```python
from build123d import *

# Parameters (mm, degrees)
CROQUIS1_R                                           = 12.5
SALIENTE_EXTRUIR1_DEPTH                              = 3.5
TALADRO_DE_MARGEN_PARA_M31_D                         = 3.4
REFRENTADO_PARA_TORNILLO_TAP_N_CON_CABEZ_D           = 3.4
REFRENTADO_PARA_TORNILLO_TAP_N_CON_CABEZ_CSINK_D     = 6.72
REFRENTADO_PARA_TORNILLO_TAP_N_CON_CABEZ_CSINK_ANGLE = 90
SALIENTE_EXTRUIR2_START                              = -29
SALIENTE_EXTRUIR2_DEPTH                              = 29
SALIENTE_EXTRUIR3_DEPTH                              = 3.5
REFRENTADO_PARA_TORNILLO_CON_CABEZA_TRON_D           = 3.4
REFRENTADO_PARA_TORNILLO_CON_CABEZA_TRON_CBORE_D     = 7
REFRENTADO_PARA_TORNILLO_CON_CABEZA_TRON_CBORE_DEPTH = 2.4


with BuildPart() as part:
    # Croquis1 → Saliente-Extruir1 (new body)
    with BuildSketch(Plane(origin=(0, 0, 0), x_dir=(0, 0, -1), z_dir=(1, 0, 0))):
        with BuildLine():
            Line((-15, 40), (-15, 29.05666877))
            ThreePointArc((-15, 29.05666877), (0, -32.7), (15, 29.05666877))
            Line((15, 29.05666877), (15, 40))
            Line((15, 40), (32.5, 40))
            ThreePointArc((32.5, 40), (47.5, 55), (32.5, 70))
            Line((32.5, 70), (-32.5, 70))
            ThreePointArc((-32.5, 70), (-47.5, 55), (-32.5, 40))
            Line((-32.5, 40), (-15, 40))
        make_face()
        Circle(CROQUIS1_R, mode=Mode.SUBTRACT)
        with BuildLine():
            Line((-32.5, 67.5), (32.5, 67.5))
            ThreePointArc((32.5, 67.5), (45, 55), (32.5, 42.5))
            Line((32.5, 42.5), (-32.5, 42.5))
            ThreePointArc((-32.5, 42.5), (-45, 55), (-32.5, 67.5))
        make_face(mode=Mode.SUBTRACT)
    extrude(amount=SALIENTE_EXTRUIR1_DEPTH)

    # Taladro de margen para M31 (through all)
    with Locations(Plane(origin=(3.5, 0, 0), x_dir=(0, 0, -1), z_dir=(1, 0, 0))):
        with Locations((0, 29), (25.11473671, 14.5), (25.11473671, -14.5), (0, -29), (-25.11473671, -14.5), (-25.11473671, 14.5)):
            Hole(TALADRO_DE_MARGEN_PARA_M31_D / 2)

    # Refrentado para tornillo tapón con cabeza plana de clavija de M31 (through all)
    with Locations(Plane(origin=(3.5, 0, 0), x_dir=(0, 0, -1), z_dir=(1, 0, 0))):
        with Locations((12.374368671, 12.374368671), (-12.374368671, -12.374368671), (-12.374368671, 12.374368671), (12.374368671, -12.374368671)):
            CounterSinkHole(REFRENTADO_PARA_TORNILLO_TAP_N_CON_CABEZ_D / 2, REFRENTADO_PARA_TORNILLO_TAP_N_CON_CABEZ_CSINK_D / 2, counter_sink_angle=REFRENTADO_PARA_TORNILLO_TAP_N_CON_CABEZ_CSINK_ANGLE)

    # Croquis8 → Saliente-Extruir2 (add)
    with BuildSketch(Plane(origin=(3.5, 0, 0), x_dir=(0, 0, -1), z_dir=(1, 0, 0)).offset(SALIENTE_EXTRUIR2_START)):
        with BuildLine():
            Line((15, 40), (32.5, 40))
            ThreePointArc((32.5, 40), (47.5, 55), (32.5, 70))
            Line((32.5, 70), (-32.5, 70))
            ThreePointArc((-32.5, 70), (-47.5, 55), (-32.5, 40))
            Line((-32.5, 40), (-15, 40))
            Line((-15, 40), (15, 40))
        make_face()
        with BuildLine():
            Line((-32.5, 67.5), (32.5, 67.5))
            ThreePointArc((32.5, 67.5), (45, 55), (32.5, 42.5))
            Line((32.5, 42.5), (-32.5, 42.5))
            ThreePointArc((-32.5, 42.5), (-45, 55), (-32.5, 67.5))
        make_face(mode=Mode.SUBTRACT)
    extrude(amount=SALIENTE_EXTRUIR2_DEPTH)

    # Croquis12 → Saliente-Extruir3 (add)
    with BuildSketch(Plane.ZY.offset(25.5)):
        with BuildLine():
            Line((32.5, 42.5), (-32.5, 42.5))
            ThreePointArc((-32.5, 42.5), (-45, 55), (-32.5, 67.5))
            Line((-32.5, 67.5), (32.5, 67.5))
            ThreePointArc((32.5, 67.5), (45, 55), (32.5, 42.5))
        make_face()
    extrude(amount=-SALIENTE_EXTRUIR3_DEPTH)

    # Refrentado para tornillo con cabeza troncocónica de M31 (through all)
    with Locations(Plane.ZY.offset(25.5)):
        with Locations((-22.5, 55), (22.5, 55)):
            CounterBoreHole(REFRENTADO_PARA_TORNILLO_CON_CABEZA_TRON_D / 2, REFRENTADO_PARA_TORNILLO_CON_CABEZA_TRON_CBORE_D / 2, REFRENTADO_PARA_TORNILLO_CON_CABEZA_TRON_CBORE_DEPTH)


solid = part.part
```
The listing builds one solid part. Answer for the finished solid, in the listing's coordinates (mm). A direction names the side the tool comes from. Coordinates: 2 decimals unless noted, no trailing zeros. Write each loop counter-clockwise with the first axis right and the second up, starting at its lowest first coordinate (ties: lowest second). Pieces come first, ordered by that corner, then holes. Notation, with made-up numbers: M 19,59.25 L 45,59.25 A9 cw 45,70.25 Z; hole C 51,76 d1. An arc over 180 degrees is marked long. Use a Markdown table: item, result. Add a question column.
1. Section D-D (y = 0) is taken. Give the vertices of the cut face in (x, z).
2. Which of the six approach directions +Z, -Z, +X, -X, +Y, -Y give full straight-line access (tool end or side, diameter ignored) to faces 4 (the flat face through (-23.1, 53, 22)), 5 (the flat face through (2, 35, 15)), 6 (the flat face through (2, 34, -15)), 7 (the cylindrical face through (-9, 55, -45))?
3. Given P1, Ø3, axis at x = 1.5, y = 32, coming from the +Z side; P2, Ø3, axis at y = 12.37, z = 12.37, coming from the +X side; P3, Ø13, axis at x = -5, z = -9, coming from the -Y side; P4, Ø5.5, axis at y = 14.5, z = 25.11, coming from the -X side, each flat-ended and moving along its own axis, determine where each tip first touches the part or whether it passes through.
4. Section B-B (x = -20.5) is taken. Give the vertices of the cut face in (y, z).
5. Section C-C (z = 0) is taken. Give the vertices of the cut face in (x, y), plus the area to 3 significant figures.
6. Straight lines are drawn through the part: line 1 along Y through (x, z) = (-22.2, -22.5); line 2 along Z through (x, y) = (-22.25, 56.5); line 3 along Y through (x, z) = (-1, -12). For each, find the intervals that lie inside material, in ascending order. Write a range as [from, to].
7. Section A-A (y = 55) is taken. Give the vertices of the cut face in (x, z).
8. For a pull along Z with two mould halves and no side action, classify faces 1 (the flat face through (3.5, 19, 1)), 2 (the cylindrical face through (-24.32, 57.95, 24.38)), 3 (the cylindrical face through (-11.203, 55.33, 47.496)) as +Z half, -Z half, draft (parallel to the pull), parting line (faces both ways), or undercut.
Data:
| question | item | result |
|---|---|---|
| 1 | outline | M 0,-32.7 L 3.5,-32.7 L 3.5,-12.5 L 0,-12.5 Z; M 0,12.5 L 3.5,12.5 L 3.5,32.7 L 0,32.7 Z |
| 2 | face 4 | -X |
| 2 | face 5 | +Z, +X, -X |
| 2 | face 6 | -Z, +X, -X |
| 2 | face 7 | +X |
| 3 | P1 | stops at z = 15 |
| 3 | P2 | passes through |
| 3 | P3 | stops at y = -32.34 |
| 3 | P4 | stops at x = 0 |
| 4 | outline | M 40,-32.5 A15 ccw 70,-32.5 L 70,32.5 A15 ccw 40,32.5 Z; hole M 42.5,-32.5 A12.5 ccw 67.5,-32.5 L 67.5,32.5 A12.5 ccw 42.5,32.5 Z |
| 5 | outline | M -25.5,40 L 0,40 L 0,30.7 L 3.5,30.7 L 3.5,42.5 L -22,42.5 L -22,67.5 L 3.5,67.5 L 3.5,70 L -25.5,70 Z; M 0,-32.7 L 3.5,-32.7 L 3.5,-30.7 L 0,-30.7 Z; M 0,-27.3 L 3.5,-27.3 L 3.5,-12.5 L 0,-12.5 Z; M 0,12.5 L 3.5,12.5 L 3.5,27.3 L 0,27.3 Z |
| 5 | area | 376 mm2 |
| 6 | line 1 | y = [40, 53.3], [56.7, 70] |
| 6 | line 2 | z = [-47.42, -23.3], [-21.7, 21.7], [23.3, 47.42] |
| 6 | line 3 | y = [40, 42.5], [67.5, 70] |
| 7 | outline | M -25.5,-47.5 L 3.5,-47.5 L 3.5,-45 L -22,-45 L -22,-24.2 L -23.1,-24.2 L -23.1,-26 L -25.5,-26 Z; M -25.5,-19 L -23.1,-19 L -23.1,-20.8 L -22,-20.8 L -22,20.8 L -23.1,20.8 L -23.1,19 L -25.5,19 Z; M -25.5,26 L -23.1,26 L -23.1,24.2 L -22,24.2 L -22,45 L 3.5,45 L 3.5,47.5 L -25.5,47.5 Z |
| 8 | face 1 | draft |
| 8 | face 2 | undercut |
| 8 | face 3 | +Z half |
